```python
from build123d import *

# Parameters (mm, degrees)
F1_DEPTH = 10


with BuildPart() as f1:
    # F0 (on Top) → F1 (new body)
    with BuildSketch(Plane.XY):
        with BuildLine():
            Line((20, 8), (-20, 8))
            Line((-20, 8), (-20, 1.7))
            ThreePointArc((-20, 1.7), (-18.797918, 1.202082), (-18.3, 0))
            ThreePointArc((-18.3, 0), (-18.797918, -1.202082), (-20, -1.7))
            Line((-20, -1.7), (-20, -8))
            Line((-20, -8), (20, -8))
            Line((20, -8), (20, -1.7))
            ThreePointArc((20, -1.7), (18.3, 0), (20, 1.7))
            Line((20, 1.7), (20, 8))
        make_face()
        with BuildLine():
            Line((-20, 1.7), (-20, 8))
            ThreePointArc((-20, 8), (-28, 0), (-20, -8))
            Line((-20, -8), (-20, -1.7))
            ThreePointArc((-20, -1.7), (-21.7, 0), (-20, 1.7))
        make_face()
        with BuildLine():
            ThreePointArc((20, -8), (28, 0), (20, 8))
            Line((20, 8), (20, 1.7))
            ThreePointArc((20, 1.7), (21.202082, 1.202082), (21.7, 0))
            ThreePointArc((21.7, 0), (21.202082, -1.202082), (20, -1.7))
            Line((20, -1.7), (20, -8))
        make_face()
    extrude(amount=F1_DEPTH)


solid = f1.part
```
Model file for the job. Use its own axes, mm. Round coordinates to 2 decimals unless told otherwise and drop trailing zeros. Write each loop counter-clockwise with the first axis right and the second up, starting at its lowest first coordinate (ties: lowest second). Pieces come first, ordered by that corner, then holes. Notation, with made-up numbers: (-22, -37.75) - (-1, -37.75) arc R31 cw to (-1, -3.75) - close; hole circle Ø6 at (-29.75, 48). An arc over 180 degrees is marked (long way). Use CSV: the item, a comma, the result in double quotes. Start each with the question number.
Item 1: Drill centre lines: L1, parallel to X at y = 1.5, z = 2; L2, parallel to Y at x = 20, z = 4.5; L3, parallel to X at y = 3.5, z = 3.75. Where is each one in solid material? Low to high. Write a range as [from, to].
Item 2: Band-saw the part on C-C (x = 19.5). Write the cut outline in (y, z).
Item 3: Pin check, flat tips, straight feed: P1, Ø1, axis at y = 6.5, z = 3.5, coming from the +X side; P2, Ø3, axis at y = 5.5, z = 6.5, coming from the -X side. Stop position of each tip, or through.
Item 4: Band-saw the part on A-A (y = 1). Write the cut outline in (x, z), and give its area (3 significant figures).
Item 5: Band-saw the part on D-D (y = 4). Write the cut outline in (x, z).
Item 6: Band-saw the part on B-B (z = 7). Write the cut outline in (x, y).
Checked values:
1,L1,"x = [-27.86, -20.8], [-19.2, 19.2], [20.8, 27.86]"
1,L2,"y = [-8, -1.7], [1.7, 8]"
1,L3,"x = [-27.19, 27.19]"
2,outline,"(-8, 0) - (-1.62, 0) - (-1.62, 10) - (-8, 10) - close; (1.62, 0) - (8, 0) - (8, 10) - (1.62, 10) - close"
3,P1,"stops at x = 25.29"
3,P2,"stops at x = -26.93"
4,outline,"(-27.94, 0) - (-21.37, 0) - (-21.37, 10) - (-27.94, 10) - close; (-18.63, 0) - (18.63, 0) - (18.63, 10) - (-18.63, 10) - close; (21.37, 0) - (27.94, 0) - (27.94, 10) - (21.37, 10) - close"
4,area,"504 mm²"
5,outline,"(-26.93, 0) - (26.93, 0) - (26.93, 10) - (-26.93, 10) - close"
6,outline,"(-20, -8) - (20, -8) arc R8 ccw to (20, 8) - (-20, 8) arc R8 ccw to start; hole (-20, -1.7) arc R1.7 ccw to (-18.3, 0) arc R1.7 ccw to (-20, 1.7) arc R1.7 ccw to start; hole (20, -1.7) arc R1.7 ccw to (21.7, 0) arc R1.7 ccw to (20, 1.7) arc R1.7 ccw to start"
